Could you check a few things on this model? Use its own coordinates, in mm. Face numbers are marked on the shaded views. A direction names the side the tool comes from. Round coordinates to 2 decimals unless told otherwise and drop trailing zeros. Loops run counter-clockwise (first coordinate to the right, second up) from the corner with the lowest first, then second, coordinate; pieces in that order, holes last. Notation, with made-up numbers: M 32.5,38 L 52.5,38 A12 ccw 52.5,61 Z; hole C 77,5.25 d10. An arc over 180 degrees is marked long. Return JSON: item names as keys, results as strings. Group by question number.
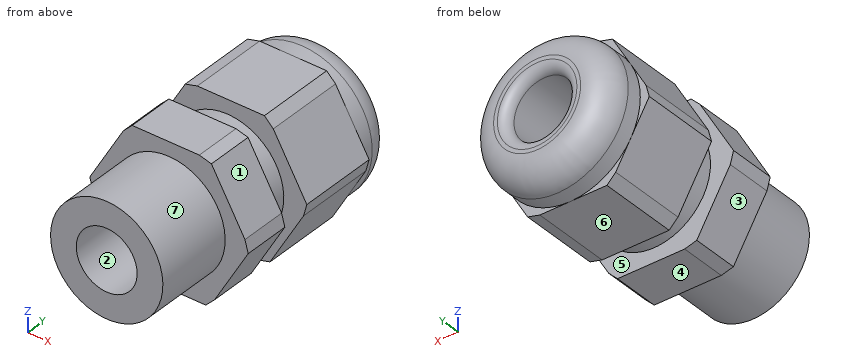
```python
from build123d import *
from OCP.BRepFilletAPI import BRepFilletAPI_MakeChamfer

# Parameters (mm, degrees)
BOSS_EXTRUDE1_DEPTH = 8.5
SKETCH4_R           = 6
BOSS_EXTRUDE2_DEPTH = 3
BOSS_EXTRUDE3_DEPTH = 5
SKETCH6_R           = 6
BOSS_EXTRUDE4_DEPTH = 8.5
SKETCH3_R           = 3.25
CUT_EXTRUDE1_DEPTH  = 32.646484797
FILLET1_R           = 1
CHAMFER1_SIZE       = 0.4
CHAMFER1_SIZE2      = 1.092820323


with BuildPart() as part:
    # Sketch1 → Boss-Extrude1 (new body)
    with BuildSketch(Plane(origin=(0, 0, 0), x_dir=(1, 0, 0), z_dir=(0, 1, 0))):
        Polygon((8.660254038, 0), (4.330127019, 7.5), (-4.330127019, 7.5), (-8.660254038, 0), (-4.330127019, -7.5), (4.330127019, -7.5), align=None)
    extrude(amount=BOSS_EXTRUDE1_DEPTH)

    # Sketch2 → Revolve1 (revolve)
    with BuildSketch(Plane(origin=(0, 0, 0), x_dir=(0, 0, -1), z_dir=(1, 0, 0))):
        with BuildLine():
            Line((-7.5, 8.5), (-7.5, 10.15))
            ThreePointArc((-7.5, 10.15), (-6.665254326, 12.165254326), (-4.65, 13))
            Line((-4.65, 13), (0, 13))
            Line((0, 13), (0, 8.5))
            Line((0, 8.5), (-7.5, 8.5))
        make_face()
    revolve(axis=Axis((0, 13, 0), (0, -1, 0)))

    # Sketch4 → Boss-Extrude2 (add)
    with BuildSketch(Plane(origin=(0, 0, 0), x_dir=(1, 0, 0), z_dir=(0, 1, 0))):
        with Locations(Location((0, 0, 0), (0, 0, 270))):
            Circle(SKETCH4_R)
    extrude(amount=-BOSS_EXTRUDE2_DEPTH)

    # Sketch5 → Boss-Extrude3 (add)
    with BuildSketch(Plane.XZ.offset(3)):
        Polygon((8.660254038, 0), (4.330127019, 7.5), (-4.330127019, 7.5), (-8.660254038, 0), (-4.330127019, -7.5), (4.330127019, -7.5), align=None)
    extrude(amount=BOSS_EXTRUDE3_DEPTH)

    # Sketch6 → Boss-Extrude4 (add)
    with BuildSketch(Plane.XZ.offset(8)):
        with Locations(Location((0, 0, 0), (0, 0, 90))):
            Circle(SKETCH6_R)
    extrude(amount=BOSS_EXTRUDE4_DEPTH)

    # Sketch3 → Cut-Extrude1 (cut, through all)
    with BuildSketch(Plane(origin=(0, 13, 0), x_dir=(1, 0, 0), z_dir=(0, 1, 0))):
        with Locations(Location((0, 0, 0), (0, 0, 270))):
            Circle(SKETCH3_R)
    extrude(amount=-CUT_EXTRUDE1_DEPTH, mode=Mode.SUBTRACT)

    # Fillet1
    fillet1_edges = [part.edges().sort_by_distance(p)[0] for p in [
        (0, 13, -3.25),
    ]]
    fillet(fillet1_edges, radius=FILLET1_R)

    # Chamfer1: one chamfer whose edges measure the first distance from different faces: ONE call of the kernel's chamfer builder (chamfer() names one face for all edges)
    chamfer1_edges_1 = [part.edges().sort_by_distance(p)[0] for p in [
        (4.330127019, 4.25, 7.5),
    ]]
    chamfer1_side_1 = [part.faces().sort_by_distance(p)[0] for p in [
        (0, 4.25, 7.5),
    ]]
    chamfer1_edges_2 = [part.edges().sort_by_distance(p)[0] for p in [
        (-4.330127019, 4.25, 7.5),
    ]]
    chamfer1_side_2 = [part.faces().sort_by_distance(p)[0] for p in [
        (-6.495190528, 4.25, 3.75),
    ]]
    chamfer1_edges_3 = [part.edges().sort_by_distance(p)[0] for p in [
        (-8.660254038, 4.25, 0),
    ]]
    chamfer1_side_3 = [part.faces().sort_by_distance(p)[0] for p in [
        (-6.495190528, 4.25, -3.75),
    ]]
    chamfer1_edges_4 = [part.edges().sort_by_distance(p)[0] for p in [
        (-4.330127019, 4.25, -7.5),
    ]]
    chamfer1_side_4 = [part.faces().sort_by_distance(p)[0] for p in [
        (0, 4.25, -7.5),
    ]]
    chamfer1_edges_5 = [part.edges().sort_by_distance(p)[0] for p in [
        (4.330127019, 4.25, -7.5),
    ]]
    chamfer1_side_5 = [part.faces().sort_by_distance(p)[0] for p in [
        (6.495190528, 4.25, -3.75),
    ]]
    chamfer1_edges_6 = [part.edges().sort_by_distance(p)[0] for p in [
        (8.660254038, 4.25, 0),
    ]]
    chamfer1_side_6 = [part.faces().sort_by_distance(p)[0] for p in [
        (6.495190528, 4.25, 3.75),
    ]]
    chamfer1_edges_7 = [part.edges().sort_by_distance(p)[0] for p in [
        (4.330127019, -5.5, -7.5),
    ]]
    chamfer1_side_7 = [part.faces().sort_by_distance(p)[0] for p in [
        (0, -5.5, -7.5),
    ]]
    chamfer1_edges_8 = [part.edges().sort_by_distance(p)[0] for p in [
        (8.660254038, -5.5, 0),
    ]]
    chamfer1_side_8 = [part.faces().sort_by_distance(p)[0] for p in [
        (6.495190528, -5.5, -3.75),
    ]]
    chamfer1_edges_9 = [part.edges().sort_by_distance(p)[0] for p in [
        (4.330127019, -5.5, 7.5),
    ]]
    chamfer1_side_9 = [part.faces().sort_by_distance(p)[0] for p in [
        (6.495190528, -5.5, 3.75),
    ]]
    chamfer1_edges_10 = [part.edges().sort_by_distance(p)[0] for p in [
        (-4.330127019, -5.5, 7.5),
    ]]
    chamfer1_side_10 = [part.faces().sort_by_distance(p)[0] for p in [
        (0, -5.5, 7.5),
    ]]
    chamfer1_edges_11 = [part.edges().sort_by_distance(p)[0] for p in [
        (-8.660254038, -5.5, 0),
    ]]
    chamfer1_side_11 = [part.faces().sort_by_distance(p)[0] for p in [
        (-6.495190528, -5.5, 3.75),
    ]]
    chamfer1_edges_12 = [part.edges().sort_by_distance(p)[0] for p in [
        (-4.330127019, -5.5, -7.5),
    ]]
    chamfer1_side_12 = [part.faces().sort_by_distance(p)[0] for p in [
        (-6.495190528, -5.5, -3.75),
    ]]
    chamfer1 = BRepFilletAPI_MakeChamfer(part.part.solid().wrapped)
    for e in chamfer1_edges_1:
        chamfer1.Add(CHAMFER1_SIZE, CHAMFER1_SIZE2, e.wrapped, chamfer1_side_1[0].wrapped)  # the first distance lies on this face
    for e in chamfer1_edges_2:
        chamfer1.Add(CHAMFER1_SIZE, CHAMFER1_SIZE2, e.wrapped, chamfer1_side_2[0].wrapped)  # the first distance lies on this face
    for e in chamfer1_edges_3:
        chamfer1.Add(CHAMFER1_SIZE, CHAMFER1_SIZE2, e.wrapped, chamfer1_side_3[0].wrapped)  # the first distance lies on this face
    for e in chamfer1_edges_4:
        chamfer1.Add(CHAMFER1_SIZE, CHAMFER1_SIZE2, e.wrapped, chamfer1_side_4[0].wrapped)  # the first distance lies on this face
    for e in chamfer1_edges_5:
        chamfer1.Add(CHAMFER1_SIZE, CHAMFER1_SIZE2, e.wrapped, chamfer1_side_5[0].wrapped)  # the first distance lies on this face
    for e in chamfer1_edges_6:
        chamfer1.Add(CHAMFER1_SIZE, CHAMFER1_SIZE2, e.wrapped, chamfer1_side_6[0].wrapped)  # the first distance lies on this face
    for e in chamfer1_edges_7:
        chamfer1.Add(CHAMFER1_SIZE, CHAMFER1_SIZE2, e.wrapped, chamfer1_side_7[0].wrapped)  # the first distance lies on this face
    for e in chamfer1_edges_8:
        chamfer1.Add(CHAMFER1_SIZE, CHAMFER1_SIZE2, e.wrapped, chamfer1_side_8[0].wrapped)  # the first distance lies on this face
    for e in chamfer1_edges_9:
        chamfer1.Add(CHAMFER1_SIZE, CHAMFER1_SIZE2, e.wrapped, chamfer1_side_9[0].wrapped)  # the first distance lies on this face
    for e in chamfer1_edges_10:
        chamfer1.Add(CHAMFER1_SIZE, CHAMFER1_SIZE2, e.wrapped, chamfer1_side_10[0].wrapped)  # the first distance lies on this face
    for e in chamfer1_edges_11:
        chamfer1.Add(CHAMFER1_SIZE, CHAMFER1_SIZE2, e.wrapped, chamfer1_side_11[0].wrapped)  # the first distance lies on this face
    for e in chamfer1_edges_12:
        chamfer1.Add(CHAMFER1_SIZE, CHAMFER1_SIZE2, e.wrapped, chamfer1_side_12[0].wrapped)  # the first distance lies on this face
    add(Compound.cast(chamfer1.Shape()), mode=Mode.REPLACE)


solid = part.part
```
1. If we section it at C-C, the plane y = -2: Please give me the cut outline in (x, z), then the cut area to 3 significant figures.
2. I'm going to push flat-ended pins straight in: pin 1 Ø3 at (x, z) = (3, -6) entering from +Y; pin 2 Ø3 at (x, z) = (-0.5, 3) entering from -Y; pin 3 Ø1.9 at (x, z) = (4.5, 5) entering from +Y; pin 4 Ø1 at (y, z) = (-13.5, 6) entering from +X. Where does each tip first touch, or does it pass through?
3. I need wall thicknesses on probe 1 along X at (y, z) = (-9.75, 0); probe 2 along Z at (x, y) = (0.25, 7.5); probe 3 along Z at (x, y) = (-2.5, 10.25). Which ranges of each line are inside material? Lowest first, please.
4. We'd pull the mould along X, two halves only. Please class the marked faces 1, 2, 3 and 4: +X half, -X half, draft (parallel to the pull), parting line (faces both ways), or undercut.
5. If we section it at B-B, the plane z = 0: Please give me the cut outline in (x, y), then the cut area to 3 significant figures.
6. On a 3-axis mill with a long thin cutter (end or side, diameter ignored), from which of +Z, -Z, +X, -X, +Y, -Y can I reach the whole of each face in a straight line? I mean the marked faces 5, 6 and 7. Say none if no direction works.
7. If we section it at A-A, the plane y = 6.75: Please give me the cut outline in (x, z).
Geometry results:
{
 "1": {"outline": "C 0,0 d12; hole C 0,0 d6.5", "area": "79.9 mm^2"},
 "2": {"pin 1": "y = 12.94", "pin 2": "y = -16.5", "pin 3": "y = 12.77", "pin 4": "x = 2.4"},
 "3": {"probe 1": "-6 to -3.25, 3.25 to 6", "probe 2": "-7.5 to -3.24, 3.24 to 7.5", "probe 3": "-7.07 to -2.08, 2.08 to 7.07"},
 "4": {"face 1": "+X half", "face 2": "undercut", "face 3": "-X half", "face 4": "draft"},
 "5": {"outline": "M -8.37,-8 L -6,-8 L -6,-16.5 L -3.25,-16.5 L -3.25,12 A1 ccw -4.25,13 L -4.65,13 A2.85 ccw -7.5,10.15 L -7.5,8.5 L -8.37,8.5 L -8.37,0 L -6,0 L -6,-3 L -8.37,-3 Z; M 3.25,-16.5 L 6,-16.5 L 6,-8 L 8.37,-8 L 8.37,-3 L 6,-3 L 6,0 L 8.37,0 L 8.37,8.5 L 7.5,8.5 L 7.5,10.15 A2.85 ccw 4.65,13 L 4.25,13 A1 ccw 3.25,12 Z", "area": "236 mm^2"},
 "6": {"face 5": "none", "face 6": "-Z, +X, -X, +Y, -Y", "face 7": "-Y"},
 "7": {"outline": "M -8.46,-0.35 L -4.88,-6.55 L -3.93,-7.5 L 3.24,-7.5 L 4.53,-7.15 L 8.11,-0.95 L 8.46,0.35 L 4.88,6.55 L 3.93,7.5 L -3.24,7.5 L -4.53,7.15 L -8.11,0.95 Z; hole C 0,0 d6.5"}
}
